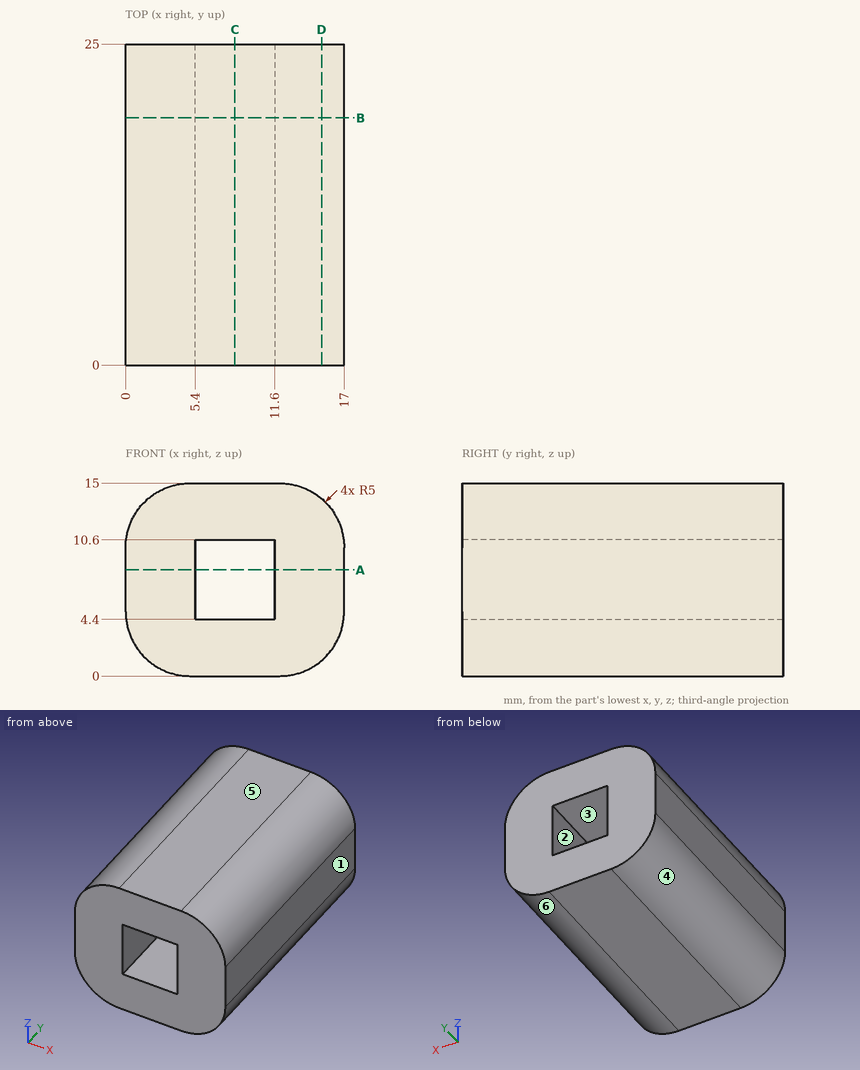
Geometry check sheet. Reference: drawing and pictorial views, mm from the part's lowest x, y, z. A direction names the side the tool comes from. Round coordinates to 2 decimals unless told otherwise and drop trailing zeros. Loops run counter-clockwise (first coordinate to the right, second up) from the corner with the lowest first, then second, coordinate; pieces in that order, holes last. Notation, with made-up numbers: (29.25, -38.75) - (38.25, -38.75) arc R23 ccw to (38.25, -23.75) - close; hole circle Ø8 at (13, -37.75). An arc over 180 degrees is marked (long way). One line per question, with ' | ' between items. Start each with the question number.
1. Scan lines: line 1 (Z direction, x = 9.75, y = 3); line 2 (X direction, y = 10.5, z = 5); line 3 (X direction, y = 8, z = 12). Record each from-to range of solid material in increasing order. Write a range as [from, to].
2. Cross-section at B-B on y = 19.25. Record the cut outline in (x, z), then the cut area to 3 significant figures.
3. Cross-section at C-C on x = 8.5. Record the cut outline in (y, z), then the cut area to 3 significant figures.
4. Depth check by flat-ended pin: pin 1 (3 mm diameter, centred on y = 18.5, z = 2.5, fed in from -X). Enter the tip coordinate at first touch or a pass-through.
5. Cross-section at A-A on z = 8.25. Record the cut outline in (x, y).
6. Tool access check on the marked faces 1 and 2. Record the directions out of +Z, -Z, +X, -X, +Y, -Y that give a thin tool (end or side, any length) a straight path to the whole face; none if there is none.
7. Cross-section at D-D on x = 15.25. Record the cut outline in (y, z).
8. Draft check along X on the marked faces 3, 4, 5 and 6. Enter one of: released by +X, released by -X, zero draft, split by the parting line, or undercut.
Taken from the geometry:
1) line 1: [0, 4.4], [10.6, 15] | line 2: [0, 5.4], [11.6, 17] | line 3: [0.42, 16.58]
2) outline: (0, 5) arc R5 ccw to (5, 0) - (12, 0) arc R5 ccw to (17, 5) - (17, 10) arc R5 ccw to (12, 15) - (5, 15) arc R5 ccw to (0, 10) - close; hole (5.4, 4.4) - (11.6, 4.4) - (11.6, 10.6) - (5.4, 10.6) - close | area: 195 mm²
3) outline: (0, 0) - (25, 0) - (25, 4.4) - (0, 4.4) - close; (0, 10.6) - (25, 10.6) - (25, 15) - (0, 15) - close | area: 220 mm²
4) pin 1: x = 0.1
5) outline: (0, 0) - (5.4, 0) - (5.4, 25) - (0, 25) - close; (11.6, 0) - (17, 0) - (17, 25) - (11.6, 25) - close
6) face 1: +Z, -Z, +X, +Y, -Y | face 2: +Y, -Y
7) outline: (0, 1.2) - (25, 1.2) - (25, 13.8) - (0, 13.8) - close
8) face 3: undercut | face 4: released by -X | face 5: zero draft | face 6: released by +X
